Read the model definition and answer for the solid it produces. Units are mm, in the model's axes. A direction names the side the tool comes from. Give positions to 0.01 mm unless a question says otherwise; leave off trailing zeros. Order: outer loops, then holes, each group sorted by start corner. A loop starts at its lowest first (then second) coordinate and runs counter-clockwise, first axis right, second up. Notation, with made-up numbers: M 37,-32 L 46,-32 A6 cw 46,-25 Z; hole C 12.5,12.5 d7. An arc over 180 degrees is marked long. One line per item, written item: value.
from build123d import *

# Parameters (mm, degrees)
ESQUISSE1_R        = 12.5
BOSS_EXTRU_1_DEPTH = 25


with BuildPart() as part:
    # Esquisse1 → Boss.-Extru.1 (new, symmetric)
    with BuildSketch(Plane.XY):
        with BuildLine():
            Line((83.869153377, -119.714830661), (93.869153377, -102.394322585))
            Line((93.869153377, -102.394322585), (41.907629149, -72.394322585))
            Line((41.907629149, -72.394322585), (35.151654556, -84.096013836))
            ThreePointArc((35.151654556, -84.096013836), (-13.596595867, -165.15744642), (-24.048474301, -259.168647929))
            ThreePointArc((-24.048474301, -259.168647929), (2.80386651, -283.348755554), (29.65620732, -259.168647929))
            ThreePointArc((29.65620732, -259.168647929), (47.428924329, -185.813223264), (83.869153377, -119.714830661))
        make_face()
        with Locations((2.80386651, -256.348755554)):
            Circle(ESQUISSE1_R, mode=Mode.SUBTRACT)
    extrude(amount=BOSS_EXTRU_1_DEPTH, both=True)

    # Esquisse3 → Enlèvement de matière-Révolution1 (revolve, cut)
    with BuildSketch(Plane.XY):
        Polygon((67.888391263, -87.394322585), (50.388391263, -117.705211717), (44.614888571, -107.705211717), (59.228137225, -82.394322585), align=None)
    revolve(axis=Axis((67.888391263, -87.394322585, 0), (-0.5000000000000014, -0.8660254037844379, 0)), mode=Mode.SUBTRACT)


solid = part.part
1) Find section C-C, the plane y = -156. Write down the section's boundary in (x, z), plus the area to 3 significant figures.
Reported:
outline: M -10.27,-25 L 61.04,-25 L 61.04,25 L -10.27,25 Z
area: 3,570 mm^2
2) Find section D-D, the plane x = -15. Write down the section's boundary in (y, z).
Reported:
outline: M -276.65,-25 L -169.45,-25 L -169.45,25 L -276.65,25 Z
3) Each of these flat-tipped pins is pushed along its axis until it touches: pin 1 Ø3 at (x, z) = (52.5, -15) entering from +Y; pin 2 Ø10 at (y, z) = (-97, -8) entering from +X; pin 3 Ø8 at (y, z) = (-244, 16.5) entering from +X. Where does it stop, or does it pass through?
Reported:
pin 1: stops at y = -77.64
pin 2: stops at x = 93.19
pin 3: stops at x = 32.33
4) Which of the six approach directions +Z, -Z, +X, -X, +Y, -Y give full straight-line access (tool end or side, diameter ignored) to faces 5 (the face through (52.083, -117.526, 1.057)), 6 (the face through (68.252, -87.604, 11.461))?
Reported:
face 5: none
face 6: +Z, -Z, +X, +Y
5) Find section B-B, the plane z = -12.5. Write down the section's boundary in (x, y), plus the area to 3 significant figures.
Reported:
outline: M -24.05,-259.17 A27 ccw 29.66,-259.17 A284.44 cw 83.87,-119.71 L 93.87,-102.39 L 41.91,-72.39 L 35.15,-84.1 A221.32 ccw Z; hole C 2.8,-256.35 d25
area: 12,100 mm^2
6) Consider probe 1 along X at (y, z) = (-246, -12); probe 2 along Y at (x, z) = (55, -2); probe 3 along Y at (x, z) = (3.5, 4.5). Determine where each line is inside the solid, lowest interval first.
Reported:
probe 1: x = -25.04 to -4.21, 9.81 to 31.35
probe 2: y = -168.13 to -117.46, -90.12 to -79.95
probe 3: y = -283.34 to -268.83, -243.87 to -126.95
7) Find section A-A, the plane x = -2. Write down the section's boundary in (y, z).
Reported:
outline: M -282.92,-25 L -267.89,-25 L -267.89,25 L -282.92,25 Z; M -244.81,-25 L -137.29,-25 L -137.29,25 L -244.81,25 Z
8) Determine the mould class of faces 1 (the face through (52.684, -95.254, 3.83)), 2 (the face through (88.799, -111.176, 0.35)), 3 (the face through (20, -176, -25)), 4 (the face through (8.57, -267.44, -0.35)) for opening direction X: +X half, -X half, draft (parallel to the pull), parting line (faces both ways), or undercut.
Reported:
face 1: undercut
face 2: +X half
face 3: draft
face 4: undercut
